Autodesk Inventor part; units mm, degrees
ref_plane "YZ Plane" through (0, 0, 0) normal (1, 0, 0) x (0, 1, 0)
ref_plane "XZ Plane" through (0, 0, 0) normal (0, 1, 0) x (-1, 0, 0)
ref_plane "XY Plane" through (0, 0, 0) normal (0, 0, 1) x (1, 0, 0)
sketch "Flange Sketch" plane through (0, 0, 0) normal (0, 1, 0) x (-1, 0, 0)
  circle A0 centre (0, 0) radius 927.1
  circle A1 centre (0, 0) radius 764.413
  circle A2 centre (0, 0) radius 879.475 construction
  line L0 (0, 0) -> (-53.1014, -877.8704) construction
  line L1 (0, 0) -> (0, -879.475) construction
  dimension "outerDiam" = 1854.2
  dimension "innerDiam" = 1528.826
  dimension "boltCircle" = 1758.95
  dimension "boltOffsetAngle" = 3.462
extrude "Flange Extrusion" add sketch "Flange Sketch" along normal blind 71.628
hole "Bolt Hole" at (53.1014, 0, -877.8704) direction (0, 1, 0) diameter 47.625 depth 71.628
pattern_circular "Bolt Hole Pattern" count 52 over 360 about axis through (0, -10, 0) along (0, 1, 0) of "Bolt Hole"
equation "\"nominalSize\" = 1524"
properties part number "AWWA C207-18 Class B Ring and Blind Flange"
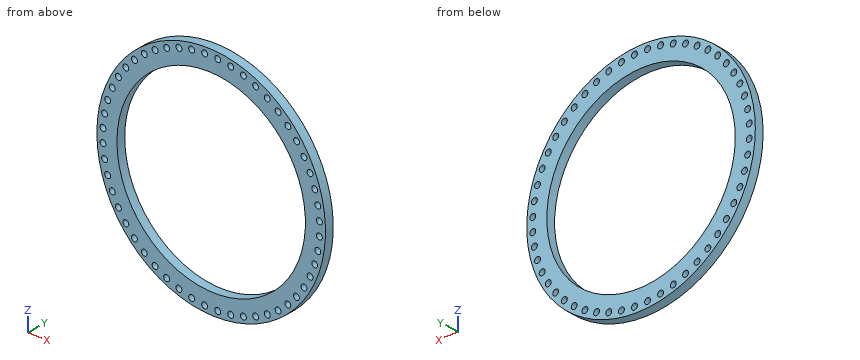
Geometry: final body of the model. Coordinates: model frame, mm. Coordinates: 2 decimals unless noted, no trailing zeros. Loops run counter-clockwise (first coordinate to the right, second up) from the corner with the lowest first, then second, coordinate; pieces in that order, holes last. Notation, with made-up numbers: (25.5, 63) - (72.5, 63) arc R23 ccw to (72.5, 87) - close; hole circle Ø9 at (64, -14). An arc over 180 degrees is marked (long way). One line per question, with ' | ' between items. Start each with the question number.
(1) Cut plane B-B on x = 0. Output: boundary loops of the cut face in (y, z), and give its area (3 significant figures).
(2) First-contact query: pin 1 (1.5 mm diameter, centred on x = 113, y = 27.5, fed in from -Z); pin 2 (12 mm diameter, centred on x = -293, y = 12.5, fed in from +Z); pin 3 (1 mm diameter, centred on y = 16, z = 572, fed in from -X). Flat tips, straight axial feed; report the tip coordinate or a pass-through.
(3) Cut plane A-A on z = 0. Output: boundary loops of the cut face in (x, y), and give its area (3 significant figures).
(4) Ray query, L1, parallel to Z at x = 155, y = 42; L2, parallel to X at y = 38.5, z = 380.5; L3, parallel to Z at x = 638.5, y = 51.5. Return the intervals inside material, ascending. Write a range as from..to.
Here are the results:
1) outline: (0, -927.1) - (71.63, -927.1) - (71.63, -764.41) - (0, -764.41) - close; (0, 764.41) - (71.63, 764.41) - (71.63, 927.1) - (0, 927.1) - close | area: 23,300 mm²
2) pin 1: z = -920.28 | pin 2: z = 881.56 | pin 3: x = -730
3) outline: (-927.1, 0) - (-764.41, 0) - (-764.41, 71.63) - (-927.1, 71.63) - close; (764.41, 0) - (927.1, 0) - (927.1, 71.63) - (764.41, 71.63) - close | area: 23,300 mm²
4) L1: -914.05..-888.62, -841.52..-748.53, 748.53..841.52, 888.62..914.05 | L2: -845.42..-815.59, -788.4..-662.98, 662.98..788.4, 815.59..845.42 | L3: -672.18..-638.94, -604.83..-420.29, 420.29..604.83, 638.94..672.18
